from build123d import *

# Parameters (mm, degrees)
SKETCH1_W               = 116
SKETCH1_H               = 115
BOSS_EXTRUDE1_DEPTH     = 4
SKETCH2_R               = 7.5
SKETCH2_R_2             = 5
BOSS_EXTRUDE2_DEPTH     = 2.5
SKETCH3_W               = 10
SKETCH3_H               = 4
BOSS_EXTRUDE3_DEPTH     = 8
SKETCH6_R               = 2.225609416
SKETCH6_R_2             = 2.302524441
CUT_EXTRUDE2_DEPTH      = 8
SKETCH7_R               = 5
BOSS_EXTRUDE5_DEPTH     = 3
SKETCH9_R               = 2
CUT_EXTRUDE3_DEPTH      = 5
CUT_EXTRUDE3_DEPTH_BACK = 8
SKETCH10_R              = 3.5
CUT_EXTRUDE5_DEPTH      = 3


with BuildPart() as part:
    # Sketch1 → Boss-Extrude1 (new body)
    with BuildSketch(Plane(origin=(0, 0, 0), x_dir=(1, 0, 0), z_dir=(0, 1, 0))):
        with Locations((-35.28313253, -23.102409639)):
            Rectangle(SKETCH1_W, SKETCH1_H)
    extrude(amount=BOSS_EXTRUDE1_DEPTH)

    # Sketch2 → Boss-Extrude2 (add)
    with BuildSketch(Plane(origin=(0, 0, 0), x_dir=(1, 0, 0), z_dir=(0, 1, 0))):
        with Locations((14.21686747, -72.602409639)):
            Circle(SKETCH2_R)
        with Locations((14.21686747, -72.602409639)):
            Circle(SKETCH2_R_2, mode=Mode.SUBTRACT)
    extrude(amount=-BOSS_EXTRUDE2_DEPTH)

    # Sketch3 → Boss-Extrude3 (add)
    with BuildSketch(Plane.ZY.offset(93.28313253)):
        with Locations((-14.397590361, 6)):
            Rectangle(SKETCH3_W, SKETCH3_H)
        with Locations((55.602409639, 6)):
            Rectangle(SKETCH3_W, SKETCH3_H)
    extrude(amount=-BOSS_EXTRUDE3_DEPTH)

    # Sketch6 → Cut-Extrude2 (cut)
    with BuildSketch(Plane.ZY.offset(93.28313253)):
        with Locations((-14.397590361, 3)):
            Circle(SKETCH6_R)
        with Locations((55.602409639, 3)):
            Circle(SKETCH6_R_2)
    extrude(amount=-CUT_EXTRUDE2_DEPTH, mode=Mode.SUBTRACT)

    # Sketch7 → Boss-Extrude5 (add)
    with BuildSketch(Plane.XZ):
        with Locations((2.71686747, -14.397590361)):
            Circle(SKETCH7_R)
    extrude(amount=BOSS_EXTRUDE5_DEPTH)

    # Sketch9 → Cut-Extrude3 (cut, two sides)
    with BuildSketch(Plane(origin=(0, 4, 0), x_dir=(1, 0, 0), z_dir=(0, 1, 0))) as cut_extrude3_sk:
        with Locations((-33.429640785, 4.397590361)):
            Circle(SKETCH9_R)
        with Locations((-33.429640785, -50.602409639)):
            Circle(SKETCH9_R)
    extrude(amount=CUT_EXTRUDE3_DEPTH, mode=Mode.SUBTRACT)
    extrude(cut_extrude3_sk.sketch, amount=-CUT_EXTRUDE3_DEPTH_BACK, mode=Mode.SUBTRACT)

    # Sketch10 → Cut-Extrude5 (cut)
    with BuildSketch(Plane.XZ):
        with Locations((-33.429640785, -4.397590361)):
            Circle(SKETCH10_R)
        with Locations((-33.429640785, 50.602409639)):
            Circle(SKETCH10_R)
    extrude(amount=-CUT_EXTRUDE5_DEPTH, mode=Mode.SUBTRACT)


solid = part.part
The listing builds one solid part. Answer for the finished solid, in the listing's coordinates (mm). A direction names the side the tool comes from. Round coordinates to 2 decimals unless told otherwise and drop trailing zeros. Write each loop counter-clockwise with the first axis right and the second up, starting at its lowest first coordinate (ties: lowest second). Pieces come first, ordered by that corner, then holes. Notation, with made-up numbers: (-4.5, 8) - (36.5, 8) arc R13 cw to (36.5, 16) - close; hole circle Ø1 at (8.5, 68). An arc over 180 degrees is marked (long way). Use one line per item in the form item = value. Start each with the question number.
Item 1: A cutting plane is placed at C-C (x = -10). Write down the section's boundary in (y, z).
Item 2: Flat-ended cylindrical pins translate along their axes: pin 1 Ø1.2 at (x, y) = (-90, 6.5) entering from -Z; pin 2 Ø1.6 at (y, z) = (1.5, -14) entering from -X; pin 3 Ø8 at (x, z) = (-27, 52) entering from -Y; pin 4 Ø1 at (x, z) = (-69, -13.5) entering from +Y. Find the tip coordinate at first contact, or state that the pin passes through.
Item 3: A tool of negligible diameter and unlimited length cuts with its end or side. For faces 1 (the cylindrical face through (-89.339, 3.101, 53.302)), 2 (the flat face through (-89, 6, -9.398)), 3 (the flat face through (-89, 6, 60.602)), 4 (the cylindrical face through (-34.188, 1.479, 47.186)), from which of +Z, -Z, +X, -X, +Y, -Y can it reach the whole face along a straight path? Write none if from no direction.
Item 4: Determine the mould class of faces 5 (the flat face through (22.717, 2, 24)), 6 (the flat face through (-36, 2, 80.602)), 7 (the flat face through (-31, 3, 51)), 8 (the cylindrical face through (16.52, -1.23, 77.04)) for opening direction Z: +Z half, -Z half, draft (parallel to the pull), parting line (faces both ways), or undercut.
Item 5: A cutting plane is placed at A-A (z = -18). Write down the section's boundary in (x, y), plus the area to 3 significant figures.
Item 6: A cutting plane is placed at B-B (x = 4). Write down the section's boundary in (y, z).
Item 7: Find the intervals of material crossed by line 1 (Y direction, x = -43, z = -20.5); line 2 (X direction, y = 6.5, z = -14), in increasing order. Write a range as [from, to].
Item 8: A cutting plane is placed at D-D (z = 36). Write down the section's boundary in (x, y), plus the area to 3 significant figures.
The answers:
q1.outline = (0, -34.4) - (4, -34.4) - (4, 80.6) - (0, 80.6) - close
q2.pin_1 = -19.4
q2.pin_2 = -93.28
q2.pin_3 = 0
q2.pin_4 = 4
q3.face_1 = -X
q3.face_2 = +X, -X, +Y
q3.face_3 = +Z, +X, -X, +Y
q3.face_4 = -Y
q4.face_5 = draft
q4.face_6 = +Z half
q4.face_7 = undercut
q4.face_8 = undercut
q5.outline = (-93.28, 0) - (-0.75, 0) - (-0.75, -3) - (6.18, -3) - (6.18, 0) - (22.72, 0) - (22.72, 4) - (-85.28, 4) - (-85.28, 8) - (-93.28, 8) - close
q5.area = 517 mm^2
q6.outline = (-3, -19.23) - (0, -19.23) - (0, -34.4) - (4, -34.4) - (4, 80.6) - (0, 80.6) - (0, -9.57) - (-3, -9.57) - close
q7.line_1 = [0, 4]
q7.line_2 = [-93.28, -85.28]
q8.outline = (-93.28, 0) - (22.72, 0) - (22.72, 4) - (-93.28, 4) - close
q8.area = 464 mm^2
